Drawing for the job (mm, zero at the part's lowest x, y, z). A direction names the side the tool comes from. Give positions to 0.01 mm unless a question says otherwise; leave off trailing zeros. Order: outer loops, then holes, each group sorted by start corner. A loop starts at its lowest first (then second) coordinate and runs counter-clockwise, first axis right, second up. Notation, with made-up numbers: (-28.75, 18) - (4.25, 18) arc R14 cw to (4.25, 29) - close; hole circle Ø1 at (76.25, 47.5). An arc over 180 degrees is marked (long way). One line per item, written item: value.
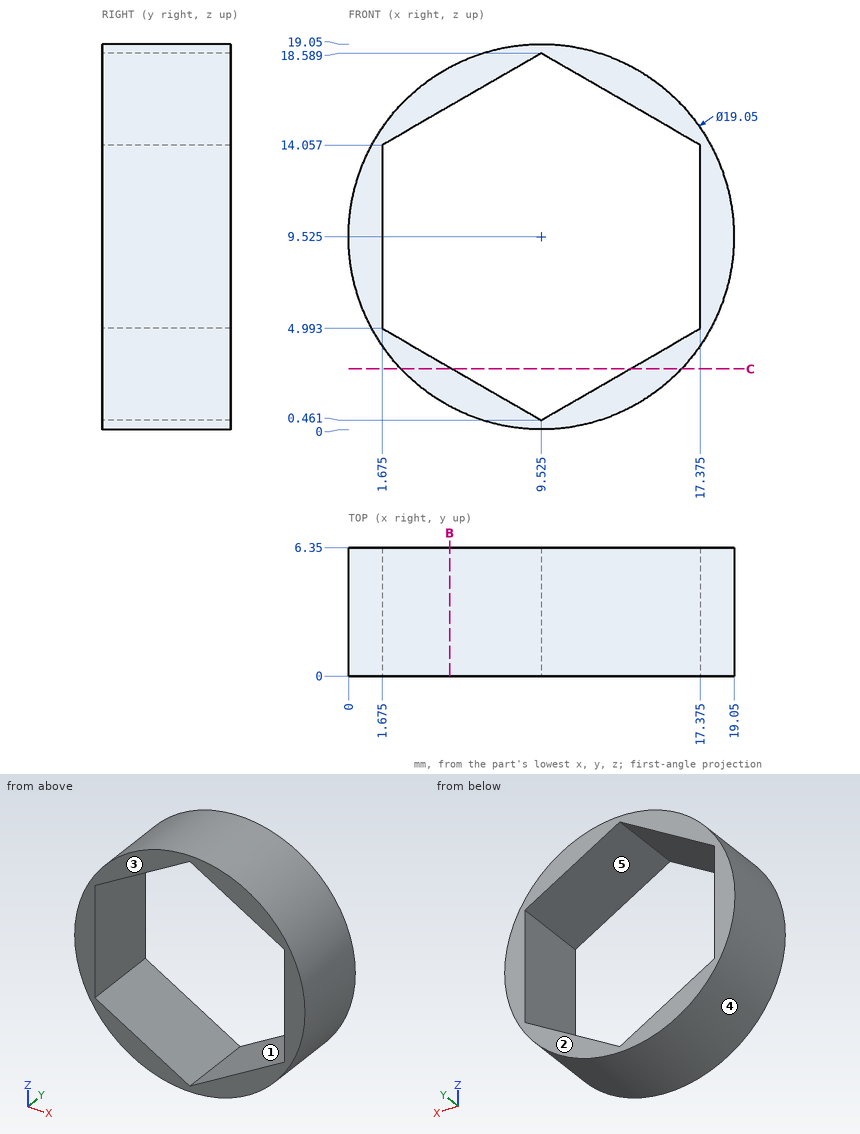
1) Mould opens along X. For the marked faces 3, 4 and 5 say: released by +X, released by -X, zero draft, split by the parting line, or undercut.
Outcome:
face 3: zero draft
face 4: split by the parting line
face 5: undercut
2) Pin check, flat tips, straight feed: pin 1 (2 mm diameter, centred on x = 16.5, y = 2.5, fed in from -Z); pin 2 (1 mm diameter, centred on y = 3.5, z = 6.5, fed in from +X); pin 3 (6 mm diameter, centred on x = 7.5, z = 4, fed in from -Y). Stop position of each tip, or through.
Outcome:
pin 1: stops at z = 2.11
pin 2: stops at x = 18.71
pin 3: stops at y = 0
3) Cut at B-B, the plane x = 5. Give the cut face in (y, z), then the cut area to 3 significant figures.
Outcome:
outline: (0, 1.14) - (6.35, 1.14) - (6.35, 3.07) - (0, 3.07) - close; (0, 15.98) - (6.35, 15.98) - (6.35, 17.91) - (0, 17.91) - close
area: 24.5 mm^2
4) Which spindle directions (+Z, -Z, +X, -X, +Y, -Y) get a long thin tool onto all of the face, cutting with end or side? Do the marked faces 1 and 2. Say none if no direction does.
Outcome:
face 1: +Y, -Y
face 2: +Z, -Z, +X, -X, +Y
5) Cut at C-C, the plane z = 3. Give the cut face in (x, y).
Outcome:
outline: (2.59, 0) - (5.13, 0) - (5.13, 6.35) - (2.59, 6.35) - close; (13.92, 0) - (16.46, 0) - (16.46, 6.35) - (13.92, 6.35) - close
6) Drill centre lines: line 1 along X through (y, z) = (0.5, 15.75) (1 decimal); line 2 along X through (y, z) = (2, 4) (1 decimal); line 3 along Z through (x, y) = (15.75, 6) (1 decimal). Where is each one in solid material? Low to high. Write a range as from..to.
Outcome:
line 1: x = 2.3..4.6, 14.4..16.7
line 2: x = 1.8..3.4, 15.7..17.3
line 3: z = 2.3..4.1, 15..16.7
